Input: part model. Units: mm. Frame: model coordinates. A direction names the side the tool comes from. Coordinates: 2 decimals unless noted, no trailing zeros. Write each loop counter-clockwise with the first axis right and the second up, starting at its lowest first coordinate (ties: lowest second). Pieces come first, ordered by that corner, then holes. Notation, with made-up numbers: M 57.5,-15 L 65.5,-15 A10 ccw 65.5,-1 Z; hole C 55.25,56.25 d8. An arc over 180 degrees is marked long. Answer as a JSON object with one key per item and string values. Group by question number.
from build123d import *

# Parameters (mm, degrees)
BOSS_EXTRUDE1_DEPTH     = 11.8
BOSS_EXTRUDE2_DEPTH     = 10.5
CUT_EXTRUDE1_DEPTH      = 18.705648816
CUT_EXTRUDE1_DEPTH_BACK = 18.705648816
SKETCH2_R               = 0.5
SKETCH5_R               = 1.1
CUT_EXTRUDE2_DEPTH      = 1
CUT_EXTRUDE3_DEPTH      = 17.597891432
CUT_EXTRUDE3_DEPTH_BACK = 17.597891432
SKETCH6_R               = 1.5


with BuildPart() as part:
    # Sketch1 → Boss-Extrude1 (new body)
    with BuildSketch(Plane(origin=(0, 0, 0), x_dir=(1, 0, 0), z_dir=(0, 1, 0))):
        Polygon((0, 0), (8, 0), (8, 2), (6, 2), (6, 7), (2, 7), (2, 2), (-2, 2), (-2, 7), (-6, 7), (-6, 2), (-8, 2), (-8, 0), align=None)
    extrude(amount=BOSS_EXTRUDE1_DEPTH)

    # Sketch4 → Boss-Extrude2 (add)
    with BuildSketch(Plane.XY):
        with BuildLine():
            Line((-2, 8.9), (-2, 2.9))
            ThreePointArc((-2, 2.9), (-4, 0.9), (-6, 2.9))
            Line((-6, 2.9), (-6, 8.9))
            ThreePointArc((-6, 8.9), (-4, 10.9), (-2, 8.9))
        make_face()
        with BuildLine():
            Line((6, 8.9), (6, 2.9))
            ThreePointArc((6, 2.9), (4, 0.9), (2, 2.9))
            Line((2, 2.9), (2, 8.9))
            ThreePointArc((2, 8.9), (4, 10.9), (6, 8.9))
        make_face()
    extrude(amount=-BOSS_EXTRUDE2_DEPTH)

    # Sketch2 → Cut-Extrude1 (cut, two sides: drawn at the far end of the back side and taken through both)
    with BuildSketch(Plane(origin=(0, 11.8, 0), x_dir=(1, 0, 0), z_dir=(0, 1, 0)).offset(-CUT_EXTRUDE1_DEPTH_BACK)):
        with Locations(Location((-4, 5, 0), (0, 0, 270))):
            Circle(SKETCH2_R)
        with Locations(Location((4, 5, 0), (0, 0, 270))):
            Circle(SKETCH2_R)
    extrude(amount=CUT_EXTRUDE1_DEPTH + CUT_EXTRUDE1_DEPTH_BACK, mode=Mode.SUBTRACT)

    # Sketch5 → Cut-Extrude2 (cut)
    with BuildSketch(Plane(origin=(0, 0, -10.5), x_dir=(-1, 0, 0), z_dir=(0, 0, -1))):
        with Locations((4, 8.9)):
            Circle(SKETCH5_R)
        with Locations((4, 2.9)):
            Circle(SKETCH5_R)
        with Locations((-4, 2.9)):
            Circle(SKETCH5_R)
        with Locations((-4, 8.9)):
            Circle(SKETCH5_R)
    extrude(amount=-CUT_EXTRUDE2_DEPTH, mode=Mode.SUBTRACT)

    # Sketch6 → Cut-Extrude3 (cut, two sides: drawn at the far end of the back side and taken through both)
    with BuildSketch(Plane(origin=(0, 0, -2), x_dir=(-1, 0, 0), z_dir=(0, 0, -1)).offset(-CUT_EXTRUDE3_DEPTH_BACK)):
        with Locations((0, 5.9)):
            Circle(SKETCH6_R)
    extrude(amount=CUT_EXTRUDE3_DEPTH + CUT_EXTRUDE3_DEPTH_BACK, mode=Mode.SUBTRACT)


solid = part.part
Q1. Draft query along X for faces 5 (the flat face through (6, 6, -5)), 6 (the flat face through (0, 11.8, -1)), 7 (the flat face through (-4, 3, -9.5)), 8 (the flat face through (-8, 6, -1)). Return one class per face: released by +X, released by -X, zero draft, split by the parting line, or undercut.
Q2. Pin query (flat end, axial travel): pin 1 Ø1 at (y, z) = (9.5, -4.5) entering from -X; pin 2 Ø1.2 at (x, y) = (-1, 4.5) entering from -Z. Return the tip coordinate at first contact, or that it passes through.
Q3. Section D-D, the plane y = 1.5. Return the cut outline in (x, z), and give its area (3 significant figures).
Q4. Section C-C, the plane y = 5.9. Return the cut outline in (x, z).
Q5. Section B-B, the plane x = 0. Return the cut outline in (y, z).
Q6. Line query: line 1 (Y direction, x = 4, z = -9.8); line 2 (X direction, y = 5.9, z = -0.5); line 3 (X direction, y = 7.5, z = -9). Output: solid intervals per line, ascending. Write a range as from..to.
Q7. Access query for faces 1 (the flat face through (0.9, 4.5, -2)), 2 (the cylindrical face through (2.95, 3.23, -10.01)), 3 (the cylindrical face through (-4, 0.9, -8.7)), 4 (the flat face through (7, 6, -2)). Directions: +Z, -Z, +X, -X, +Y, -Y. A direction counts if a zero-diameter tool reaches every point of the face in a straight line with its end or side. Return the directions, or none.
Q8. Section A-A, the plane z = -2.5. Return the cut outline in (x, y), and give its area (3 significant figures).
Filled in:
{
 "1": {"face 5": "released by +X", "face 6": "zero draft", "face 7": "undercut", "face 8": "released by -X"},
 "2": {"pin 1": "x = -6", "pin 2": "z = -2"},
 "3": {"outline": "M -8,-2 L -6,-2 L -6,-7 L -5.43,-7 L -5.43,-10.5 L -2.57,-10.5 L -2.57,-7 L -2,-7 L -2,-2 L 2,-2 L 2,-7 L 2.57,-7 L 2.57,-10.5 L 5.43,-10.5 L 5.43,-7 L 6,-7 L 6,-2 L 8,-2 L 8,0 L -8,0 Z; hole C -4,-5 d1; hole C 4,-5 d1", "area": "90.4 mm^2"},
 "4": {"outline": "M -8,-2 L -6,-2 L -6,-10.5 L -2,-10.5 L -2,-2 L -1.5,-2 L -1.5,0 L -8,0 Z; M 1.5,-2 L 2,-2 L 2,-10.5 L 6,-10.5 L 6,-2 L 8,-2 L 8,0 L 1.5,0 Z; hole C -4,-5 d1; hole C 4,-5 d1"},
 "5": {"outline": "M 0,-2 L 4.4,-2 L 4.4,0 L 0,0 Z; M 7.4,-2 L 11.8,-2 L 11.8,0 L 7.4,0 Z"},
 "6": {"line 1": "0.9..1.8, 4..7.8, 10..10.9", "line 2": "-8..-1.5, 1.5..8", "line 3": "-6..-2, 2..6"},
 "7": {"face 1": "-Z, +Y, -Y", "face 2": "-Z", "face 3": "-Z, -Y", "face 4": "-Z, +X, +Y, -Y"},
 "8": {"outline": "M -6,0 L -2,0 L -2,11.8 L -6,11.8 Z; M 2,0 L 6,0 L 6,11.8 L 2,11.8 Z", "area": "94.4 mm^2"}
}
